Geometry check sheet. Reference: the model listing, model coordinates, mm. A direction names the side the tool comes from. Give positions to 0.01 mm unless a question says otherwise; leave off trailing zeros. Loops run counter-clockwise (first coordinate to the right, second up) from the corner with the lowest first, then second, coordinate; pieces in that order, holes last.
1. Release check for a two-part mould opening along X. For faces 5 (the flat face through (17, 3, 96.556)), 6 (the flat face through (-95, 3, -28.523)), 7 (the flat face through (16, 3, -5.114)), 8 (the cylindrical face through (144.454, 2.833, -26.35)) record: +X half, -X half, draft (parallel to the pull), parting line (faces both ways), or undercut.
2. Tool access check on faces 1 (the flat face through (-94, 3, 79.635)), 2 (the flat face through (123, 3, 79.635)), 3 (the flat face through (123, 3, -28.523)), 4 (the flat face through (17, 3, 90.556)). Record the directions out of +Z, -Z, +X, -X, +Y, -Y that give a thin tool (end or side, any length) a straight path to the whole face; none if there is none.
3. Cross-section at C-C, the plane y = 3.4. State how many separate pieces and enclosed holes the cut face has, plus the area to 3 significant figures.
4. Go/stop test with flat-tipped pins: pin 1 Ø3 at (x, z) = (-43.25, 65.04) entering from +Y; pin 2 Ø1 at (x, y) = (-67, 1) entering from -Z. Record where each tip stops, or that it passes through.
5. Cross-section at A-A, the plane z = 24.5. Record the cut outline in (x, y).
6. Material ranges on L1, parallel to Z at x = 11.5, y = 1.35; L2, parallel to Z at x = -23.5, y = 4.8; L3, parallel to Z at x = 39, y = 4.25, recorded low to high.
7. Cross-section at B-B, the plane x = -100. Record the cut outline in (y, z), plus the area to 3 significant figures.
from build123d import *

# Parameters (mm, degrees)
BOSS_EXTRUDE1_DEPTH = 5.588
SKETCH2_R           = 2.159
CUT_EXTRUDE1_DEPTH  = 158.413946399
SKETCH3_W           = 152.51
SKETCH3_H           = 61.34
CUT_EXTRUDE2_DEPTH  = 158.413946399
BOSS_EXTRUDE2_DEPTH = 5.588
BOSS_EXTRUDE3_DEPTH = 5.588
SKETCH7_R           = 1.75
CUT_EXTRUDE4_DEPTH  = 187.865769606
SKETCH9_R           = 1.75
CUT_EXTRUDE8_DEPTH  = 187.865769606
CUT_EXTRUDE9_DEPTH  = 187.865769606
FILLET1_R           = 3
SKETCH11_R          = 1.905
CUT_EXTRUDE10_DEPTH = 187.865769606


with BuildPart() as part:
    # Sketch1 → Boss-Extrude1 (new body)
    with BuildSketch(Plane(origin=(0, 0, 0), x_dir=(1, 0, 0), z_dir=(0, 1, 0))):
        Polygon((-73.254183378, 28.522688753), (-37.333158894, 64.443713237), (70.824792138, 64.443713237), (106.745816622, 28.522688753), (106.745816622, -79.635262279), (70.824792138, -115.556286763), (-37.333158894, -115.556286763), (-73.254183378, -79.635262279), align=None)
    extrude(amount=BOSS_EXTRUDE1_DEPTH)

    # Sketch2 → Cut-Extrude1 (cut, through all)
    with BuildSketch(Plane(origin=(0, 5.588, 0), x_dir=(1, 0, 0), z_dir=(0, 1, 0))):
        with Locations(Location((-48.254183378, 39.443713237, 0), (0, 0, 270))):
            Circle(SKETCH2_R)
        with Locations(Location((-30.576513848, 21.766043708, 0), (0, 0, 270))):
            Circle(SKETCH2_R)
        with Locations(Location((-48.254183378, -90.556286763, 0), (0, 0, 270))):
            Circle(SKETCH2_R)
        with Locations(Location((-30.576513848, -72.878617233, 0), (0, 0, 270))):
            Circle(SKETCH2_R)
        with Locations(Location((64.068147093, 21.766043708, 0), (0, 0, 270))):
            Circle(SKETCH2_R)
        with Locations(Location((81.745816622, 39.443713237, 0), (0, 0, 270))):
            Circle(SKETCH2_R)
        with Locations(Location((64.068147093, -72.878617233, 0), (0, 0, 270))):
            Circle(SKETCH2_R)
        with Locations(Location((81.745816622, -90.556286763, 0), (0, 0, 270))):
            Circle(SKETCH2_R)
    extrude(amount=-CUT_EXTRUDE1_DEPTH, mode=Mode.SUBTRACT)

    # Sketch3 → Cut-Extrude2 (cut, through all)
    with BuildSketch(Plane(origin=(0, 5.588, 0), x_dir=(1, 0, 0), z_dir=(0, 1, 0))):
        with Locations((16.745816622, -25.556286763)):
            Rectangle(SKETCH3_W, SKETCH3_H)
    extrude(amount=-CUT_EXTRUDE2_DEPTH, mode=Mode.SUBTRACT)

    # Sketch5 → Boss-Extrude2 (add)
    with BuildSketch(Plane(origin=(0, 5.588, 0), x_dir=(1, 0, 0), z_dir=(0, 1, 0))):
        with BuildLine():
            Line((-73.254183378, -79.635262279), (-115.634183378, -79.635262279))
            ThreePointArc((-115.634183378, -79.635262279), (-121.02233705, -77.403415951), (-123.254183378, -72.015262279))
            Line((-123.254183378, -72.015262279), (-123.254183378, 20.902688753))
            ThreePointArc((-123.254183378, 20.902688753), (-121.02233705, 26.290842426), (-115.634183378, 28.522688753))
            Line((-115.634183378, 28.522688753), (-73.254183378, 28.522688753))
            Line((-73.254183378, 28.522688753), (-73.254183378, -79.635262279))
        make_face()
    extrude(amount=-BOSS_EXTRUDE2_DEPTH)

    # Sketch6 → Boss-Extrude3 (add)
    with BuildSketch(Plane(origin=(0, 5.588, 0), x_dir=(1, 0, 0), z_dir=(0, 1, 0))):
        with BuildLine():
            Line((106.745816622, 28.522688753), (139.125816622, 28.522688753))
            ThreePointArc((139.125816622, 28.522688753), (144.513970295, 26.290842426), (146.745816622, 20.902688753))
            Line((146.745816622, 20.902688753), (146.745816622, -72.015262279))
            ThreePointArc((146.745816622, -72.015262279), (144.513970295, -77.403415951), (139.125816622, -79.635262279))
            Line((139.125816622, -79.635262279), (106.745816622, -79.635262279))
            Line((106.745816622, -79.635262279), (106.745816622, 28.522688753))
        make_face()
    extrude(amount=-BOSS_EXTRUDE3_DEPTH)

    # Sketch7 → Cut-Extrude4 (cut, through all)
    with BuildSketch(Plane(origin=(0, 5.588, 0), x_dir=(1, 0, 0), z_dir=(0, 1, 0))):
        with Locations(Location((110.045816622, -10.356286763, 0), (0, 0, 270))):
            Circle(SKETCH7_R)
        with Locations(Location((134.045816622, -10.356286763, 0), (0, 0, 270))):
            Circle(SKETCH7_R)
        with Locations(Location((110.045816622, -40.756286763, 0), (0, 0, 270))):
            Circle(SKETCH7_R)
        with Locations(Location((134.045816622, -40.756286763, 0), (0, 0, 270))):
            Circle(SKETCH7_R)
    extrude(amount=-CUT_EXTRUDE4_DEPTH, mode=Mode.SUBTRACT)

    # Sketch9 → Cut-Extrude8 (cut, through all)
    with BuildSketch(Plane(origin=(0, 5.588, 0), x_dir=(1, 0, 0), z_dir=(0, 1, 0))):
        with Locations(Location((-53.254183378, 13.923713237, 0), (0, 0, 270))):
            Circle(SKETCH9_R)
        with Locations(Location((-43.254183378, 13.923713237, 0), (0, 0, 270))):
            Circle(SKETCH9_R)
        with Locations(Location((-33.254183378, 13.923713237, 0), (0, 0, 270))):
            Circle(SKETCH9_R)
        with Locations(Location((-23.254183378, 13.923713237, 0), (0, 0, 270))):
            Circle(SKETCH9_R)
        with Locations(Location((-13.254183378, 13.923713237, 0), (0, 0, 270))):
            Circle(SKETCH9_R)
        with Locations(Location((-3.254183378, 13.923713237, 0), (0, 0, 270))):
            Circle(SKETCH9_R)
        with Locations(Location((6.745816622, 13.923713237, 0), (0, 0, 270))):
            Circle(SKETCH9_R)
        with Locations(Location((16.745816622, 13.923713237, 0), (0, 0, 270))):
            Circle(SKETCH9_R)
        with Locations(Location((26.745816622, 13.923713237, 0), (0, 0, 270))):
            Circle(SKETCH9_R)
        with Locations(Location((36.745816622, 13.923713237, 0), (0, 0, 270))):
            Circle(SKETCH9_R)
        with Locations(Location((46.745816622, 13.923713237, 0), (0, 0, 270))):
            Circle(SKETCH9_R)
        with Locations(Location((56.745816622, 13.923713237, 0), (0, 0, 270))):
            Circle(SKETCH9_R)
        with Locations(Location((66.745816622, 13.923713237, 0), (0, 0, 270))):
            Circle(SKETCH9_R)
        with Locations(Location((76.745816622, 13.923713237, 0), (0, 0, 270))):
            Circle(SKETCH9_R)
        with Locations(Location((86.745816622, 13.923713237, 0), (0, 0, 270))):
            Circle(SKETCH9_R)
        with Locations(Location((-53.254183378, -65.036286763, 0), (0, 0, 270))):
            Circle(SKETCH9_R)
        with Locations(Location((-43.254183378, -65.036286763, 0), (0, 0, 270))):
            Circle(SKETCH9_R)
        with Locations(Location((-33.254183378, -65.036286763, 0), (0, 0, 270))):
            Circle(SKETCH9_R)
        with Locations(Location((-23.254183378, -65.036286763, 0), (0, 0, 270))):
            Circle(SKETCH9_R)
        with Locations(Location((-13.254183378, -65.036286763, 0), (0, 0, 270))):
            Circle(SKETCH9_R)
        with Locations(Location((-3.254183378, -65.036286763, 0), (0, 0, 270))):
            Circle(SKETCH9_R)
        with Locations(Location((6.745816622, -65.036286763, 0), (0, 0, 270))):
            Circle(SKETCH9_R)
        with Locations(Location((16.745816622, -65.036286763, 0), (0, 0, 270))):
            Circle(SKETCH9_R)
        with Locations(Location((26.745816622, -65.036286763, 0), (0, 0, 270))):
            Circle(SKETCH9_R)
        with Locations(Location((36.745816622, -65.036286763, 0), (0, 0, 270))):
            Circle(SKETCH9_R)
        with Locations(Location((46.745816622, -65.036286763, 0), (0, 0, 270))):
            Circle(SKETCH9_R)
        with Locations(Location((56.745816622, -65.036286763, 0), (0, 0, 270))):
            Circle(SKETCH9_R)
        with Locations(Location((66.745816622, -65.036286763, 0), (0, 0, 270))):
            Circle(SKETCH9_R)
        with Locations(Location((76.745816622, -65.036286763, 0), (0, 0, 270))):
            Circle(SKETCH9_R)
        with Locations(Location((86.745816622, -65.036286763, 0), (0, 0, 270))):
            Circle(SKETCH9_R)
    extrude(amount=-CUT_EXTRUDE8_DEPTH, mode=Mode.SUBTRACT)

    # Sketch10 → Cut-Extrude9 (cut, through all)
    with BuildSketch(Plane(origin=(0, 5.588, 0), x_dir=(1, 0, 0), z_dir=(0, 1, 0))):
        with BuildLine():
            Line((11.245816622, 45.443713237), (22.245816622, 45.443713237))
            ThreePointArc((22.245816622, 45.443713237), (23.660030185, 44.8579268), (24.245816622, 43.443713237))
            Line((24.245816622, 43.443713237), (24.245816622, 41.443713237))
            ThreePointArc((24.245816622, 41.443713237), (23.660030185, 40.029499675), (22.245816622, 39.443713237))
            Line((22.245816622, 39.443713237), (11.245816622, 39.443713237))
            ThreePointArc((11.245816622, 39.443713237), (9.83160306, 40.029499675), (9.245816622, 41.443713237))
            Line((9.245816622, 41.443713237), (9.245816622, 43.443713237))
            ThreePointArc((9.245816622, 43.443713237), (9.83160306, 44.8579268), (11.245816622, 45.443713237))
        make_face()
        with BuildLine():
            Line((11.245816622, -90.556286763), (22.245816622, -90.556286763))
            ThreePointArc((22.245816622, -90.556286763), (23.660030185, -91.1420732), (24.245816622, -92.556286763))
            Line((24.245816622, -92.556286763), (24.245816622, -94.556286763))
            ThreePointArc((24.245816622, -94.556286763), (23.660030185, -95.970500325), (22.245816622, -96.556286763))
            Line((22.245816622, -96.556286763), (11.245816622, -96.556286763))
            ThreePointArc((11.245816622, -96.556286763), (9.83160306, -95.970500325), (9.245816622, -94.556286763))
            Line((9.245816622, -94.556286763), (9.245816622, -92.556286763))
            ThreePointArc((9.245816622, -92.556286763), (9.83160306, -91.1420732), (11.245816622, -90.556286763))
        make_face()
    extrude(amount=-CUT_EXTRUDE9_DEPTH, mode=Mode.SUBTRACT)

    # Fillet1
    fillet1_edges = [part.edges().sort_by_distance(p)[0] for p in [
        (-59.509183378, 2.794, 56.226286763),
        (-59.509183378, 2.794, -5.113713237),
        (93.000816622, 2.794, -5.113713237),
        (93.000816622, 2.794, 56.226286763),
    ]]
    fillet(fillet1_edges, radius=FILLET1_R)

    # Sketch11 → Cut-Extrude10 (cut, through all)
    with BuildSketch(Plane(origin=(0, 5.588, 0), x_dir=(1, 0, 0), z_dir=(0, 1, 0))):
        with Locations(Location((-108.254183378, -11.332286763, 0), (0, 0, 270))):
            Circle(SKETCH11_R)
        with Locations(Location((-80.822183378, -11.332286763, 0), (0, 0, 270))):
            Circle(SKETCH11_R)
        with Locations(Location((-80.822183378, -39.780286763, 0), (0, 0, 270))):
            Circle(SKETCH11_R)
        with Locations(Location((-108.254183378, -39.780286763, 0), (0, 0, 270))):
            Circle(SKETCH11_R)
    extrude(amount=-CUT_EXTRUDE10_DEPTH, mode=Mode.SUBTRACT)


solid = part.part
Result:
1. face 5: undercut
1. face 6: draft
1. face 7: undercut
1. face 8: +X half
2. face 1: +Z, -X, +Y, -Y
2. face 2: +Z, +X, +Y, -Y
2. face 3: -Z, +X, +Y, -Y
2. face 4: +Y, -Y
3. separate pieces: 1
3. enclosed holes: 49
3. area: 29,500 mm2
4. pin 1: passes through
4. pin 2: stops at z = -35.28
5. outline: (-123.25, 0) - (-59.51, 0) - (-59.51, 5.59) - (-123.25, 5.59) - close; (93, 0) - (146.75, 0) - (146.75, 5.59) - (93, 5.59) - close
6. L1: z = -64.44 to -45.44, -39.44 to -5.11, 56.23 to 90.56, 96.56 to 115.56
6. L2: z = -64.44 to -15.66, -12.19 to -5.11, 56.23 to 63.3, 66.77 to 115.56
6. L3: z = -64.44 to -5.11, 56.23 to 115.56
7. outline: (0, -28.52) - (5.59, -28.52) - (5.59, 79.64) - (0, 79.64) - close
7. area: 604 mm2
